Read the model definition and answer for the solid it produces. Units are mm, in the model's axes. Coordinates: 2 decimals unless noted, no trailing zeros. Write each loop counter-clockwise with the first axis right and the second up, starting at its lowest first coordinate (ties: lowest second). Pieces come first, ordered by that corner, then holes.
Item 1: Section B-B (x = -5) is taken. Give the vertices of the cut face in (y, z).
Item 2: Section A-A (y = -18) is taken. Give the vertices of the cut face in (x, z), then the cut area to 3 significant figures.
Item 3: Straight lines are drawn through the part: probe 1 along X at (y, z) = (-5, 0.4); probe 2 along Z at (x, y) = (-7, 9). For each, find the intervals that lie inside material, in ascending order.
Item 4: Each of these flat-tipped pins is pushed along its axis until it touches: P1, Ø0.6, axis at x = 3, z = 0.5, coming from the +Y side; P2, Ø0.9, axis at x = 9, z = 0.5, coming from the -Y side; P3, Ø0.6, axis at y = 3, z = 0.5, coming from the -X side. Where does it stop, or does it pass through?
Item 5: Determine the mould class of faces 1 (the face through (-20, 0, -1)), 2 (the face through (0, -32.5, -1)), 3 (the face through (0, 32.5, -1)) for opening direction Y: released by +Y, released by -Y, zero draft, split by the parting line, or undercut.
from build123d import *

# Parameters (mm, degrees)
F0_W     = 40
F0_H     = 65
F0_W_2   = 0.8
F0_H_2   = 50
F1_DEPTH = 2.5
F2_DEPTH = 0.8


with BuildPart() as f1:
    # F0 (on Top) → F1 (new body)
    with BuildSketch(Plane.XY):
        Rectangle(F0_W, F0_H)
        with Locations((-14.5, 0)):
            Rectangle(F0_W_2, F0_H_2, mode=Mode.SUBTRACT)
        with Locations((-8.7, 0)):
            Rectangle(F0_W_2, F0_H_2, mode=Mode.SUBTRACT)
        with Locations((-2.9, 0)):
            Rectangle(F0_W_2, F0_H_2, mode=Mode.SUBTRACT)
        with Locations((2.9, 0)):
            Rectangle(F0_W_2, F0_H_2, mode=Mode.SUBTRACT)
        with Locations((8.7, 0)):
            Rectangle(F0_W_2, F0_H_2, mode=Mode.SUBTRACT)
        with Locations((14.5, 0)):
            Rectangle(F0_W_2, F0_H_2, mode=Mode.SUBTRACT)
        with Locations((14.5, 0)):
            Rectangle(F0_W_2, F0_H_2)
        with Locations((8.7, 0)):
            Rectangle(F0_W_2, F0_H_2)
        with Locations((2.9, 0)):
            Rectangle(F0_W_2, F0_H_2)
        with Locations((-2.9, 0)):
            Rectangle(F0_W_2, F0_H_2)
        with Locations((-8.7, 0)):
            Rectangle(F0_W_2, F0_H_2)
        with Locations((-14.5, 0)):
            Rectangle(F0_W_2, F0_H_2)
    extrude(amount=-F1_DEPTH)

    # F0 (on Top) → F2 (join)
    with BuildSketch(Plane.XY):
        with Locations((14.5, 0)):
            Rectangle(F0_W_2, F0_H_2)
        with Locations((8.7, 0)):
            Rectangle(F0_W_2, F0_H_2)
        with Locations((2.9, 0)):
            Rectangle(F0_W_2, F0_H_2)
        with Locations((-2.9, 0)):
            Rectangle(F0_W_2, F0_H_2)
        with Locations((-8.7, 0)):
            Rectangle(F0_W_2, F0_H_2)
        with Locations((-14.5, 0)):
            Rectangle(F0_W_2, F0_H_2)
    extrude(amount=F2_DEPTH)


solid = f1.part
Established:
1. outline: (-32.5, -2.5) - (32.5, -2.5) - (32.5, 0) - (-32.5, 0) - close
2. outline: (-20, -2.5) - (20, -2.5) - (20, 0) - (14.9, 0) - (14.9, 0.8) - (14.1, 0.8) - (14.1, 0) - (9.1, 0) - (9.1, 0.8) - (8.3, 0.8) - (8.3, 0) - (3.3, 0) - (3.3, 0.8) - (2.5, 0.8) - (2.5, 0) - (-2.5, 0) - (-2.5, 0.8) - (-3.3, 0.8) - (-3.3, 0) - (-8.3, 0) - (-8.3, 0.8) - (-9.1, 0.8) - (-9.1, 0) - (-14.1, 0) - (-14.1, 0.8) - (-14.9, 0.8) - (-14.9, 0) - (-20, 0) - close
2. area: 104 mm2
3. probe 1: x = -14.9 to -14.1, -9.1 to -8.3, -3.3 to -2.5, 2.5 to 3.3, 8.3 to 9.1, 14.1 to 14.9
3. probe 2: z = -2.5 to 0
4. P1: stops at y = 25
4. P2: stops at y = -25
4. P3: stops at x = -14.9
5. face 1: zero draft
5. face 2: released by -Y
5. face 3: released by +Y
